```python
from build123d import *

# Parameters (mm, degrees)
BOSS_EXTRUDE1_DEPTH         = 9.525
F_8_32_TAPPED_HOLE1_D       = 3.4544
F_10_24_TAPPED_HOLE1_D      = 3.7973
F_1_4_20_TAPPED_HOLE1_D     = 5.1054
F_1_4_20_TAPPED_HOLE1_DEPTH = 19.05
F_1_4_20_TAPPED_HOLE1_TIP   = 1.533816902
FILLET1_R                   = 6.35


with BuildPart() as part:
    # Sketch1 → Boss-Extrude1 (new body)
    with BuildSketch(Plane(origin=(0, 0, 0), x_dir=(1, 0, 0), z_dir=(0, 1, 0))):
        Polygon((32.770273681, 9.766101756), (70.870273681, 9.766101756), (70.870273681, -41.414898244), (-56.129726319, -41.414898244), (-56.129726319, 9.766101756), (-18.029726319, 9.766101756), (-18.029726319, 60.566101756), (32.770273681, 60.566101756), align=None)
    extrude(amount=BOSS_EXTRUDE1_DEPTH)

    # #8-32 Tapped Hole1 (through all)
    with Locations(Plane(origin=(0, 9.525, 0), x_dir=(1, 0, 0), z_dir=(0, 1, 0))):
        with Locations((-47.354026319, 5.606851756), (-47.354026319, -37.255648244), (-21.954026319, -37.255648244), (-21.954026319, 5.606851756), (62.094573681, 5.606851756), (62.094573681, -37.255648244), (36.694573681, -37.255648244), (36.694573681, 5.606851756)):
            Hole(F_8_32_TAPPED_HOLE1_D / 2)

    # #10-24 Tapped Hole1 (through all)
    with Locations(Plane(origin=(0, 9.525, 0), x_dir=(1, 0, 0), z_dir=(0, 1, 0))):
        with Locations((5.058873681, 34.975601756), (17.758873681, 34.975601756), (5.058873681, 9.575601756), (17.758873681, 9.575601756)):
            Hole(F_10_24_TAPPED_HOLE1_D / 2)

    # 1/4-20 Tapped Hole1
    with Locations(Plane(origin=(0, 0, -60.566101756), x_dir=(-1, 0, 0), z_dir=(0, 0, -1))):
        with Locations((8.504726319, 4.7625), (-7.370273681, 4.7625), (-23.245273681, 4.7625)):
            Hole(F_1_4_20_TAPPED_HOLE1_D / 2, depth=F_1_4_20_TAPPED_HOLE1_DEPTH)
            with Locations((0, 0, -(F_1_4_20_TAPPED_HOLE1_DEPTH + F_1_4_20_TAPPED_HOLE1_TIP / 2))):  # 118° drill point
                Cone(0, F_1_4_20_TAPPED_HOLE1_D / 2, F_1_4_20_TAPPED_HOLE1_TIP, mode=Mode.SUBTRACT)

    # Fillet1
    fillet1_edges = [part.edges().sort_by_distance(p)[0] for p in [
        (32.770273681, 4.7625, -9.766101756),
        (-18.029726319, 4.7625, -9.766101756),
    ]]
    fillet(fillet1_edges, radius=FILLET1_R)


solid = part.part
```
Design review of the part built by this model. Coordinates are the model's own, in mm. A direction names the side the tool comes from. Give positions to 0.01 mm unless a question says otherwise; leave off trailing zeros. Write each loop counter-clockwise with the first axis right and the second up, starting at its lowest first coordinate (ties: lowest second). Pieces come first, ordered by that corner, then holes. Notation, with made-up numbers: (73.25, 38) - (92.25, 38) arc R17 ccw to (92.25, 43) - close; hole circle Ø7 at (-1.75, -28.5). An arc over 180 degrees is marked (long way). Return JSON: item names as keys, results as strings. Group by question number.
(1) Insertion check: pin 1 (3 mm diameter, centred on x = -48, y = 5.5, fed in from -Z); pin 2 (5 mm diameter, centred on y = 3.5, z = -49, fed in from -X). Each pin has a flat end and moves straight along its axis. Give the tip position at first contact, or say it passes through.
(2) To check wall thickness, follow probe 1 along X at (y, z) = (4.5, -35); probe 2 along X at (y, z) = (2.5, -56); probe 3 along Z at (x, y) = (35.5, 5.5). State the ranges of each line that lie inside material, in increasing order.
(3) We need section B-B, the plane z = -24.5. Give the boundary of the cut face in (x, y) (3 decimals), then the cut area to 3 significant figures.
(4) Mouldability with a two-part tool opening along Z and no side actions: class faces 5 (the cylindrical face through (-23.55, 4.7, 37.92)), 6 (the cylindrical face through (25.68, 5.53, -50.91)), 7 (the conical face through (-8.447, 5.202, -40.249)) as +Z half, -Z half, draft (parallel to the pull), parting line (faces both ways), or undercut.
(5) Machinability: for faces 1 (the flat face through (-18.03, 5, -38)), 2 (the cylindrical face through (9.805, 5.529, -50.908)), 3 (the flat face through (8, 5, 41.415)), 4 (the flat face through (32.77, 5, -39)), which of the approach directions +Z, -Z, +X, -X, +Y, -Y give a long, thin tool a straight path to every point of the face, cutting with its end or side? Answer none if there is none.
(6) We need section A-A, the plane z = -46. Give the boundary of the cut face in (x, y) (1 decimal).
Reported:
{
 "1": {"pin 1": "stops at z = -9.77", "pin 2": "stops at x = -18.03"},
 "2": {"probe 1": "x = -18.03 to 3.16, 6.96 to 15.86, 19.66 to 32.77", "probe 2": "x = -18.03 to -9.69, -7.32 to 6.19, 8.55 to 22.06, 24.43 to 32.77", "probe 3": "z = -10.9 to -6.85, -4.36 to 36.01, 38.5 to 41.41"},
 "3": {"outline": "(-18.03, 0) - (32.77, 0) - (32.77, 9.525) - (-18.03, 9.525) - close", "area": "484 mm2"},
 "4": {"face 5": "undercut", "face 6": "draft", "face 7": "-Z half"},
 "5": {"face 1": "-Z, -X, +Y, -Y", "face 2": "-Z", "face 3": "+Z, +X, -X, +Y, -Y", "face 4": "-Z, +X, +Y, -Y"},
 "6": {"outline": "(-18, 0) - (32.8, 0) - (32.8, 9.5) - (-18, 9.5) - close; hole circle Ø5.1 at (-8.5, 4.8); hole circle Ø5.1 at (7.4, 4.8); hole circle Ø5.1 at (23.2, 4.8)"}
}
